from build123d import *

# Parameters (mm, degrees)
SKETCH2_W               = 26
SKETCH2_H               = 6.2
BOSS_EXTRUDE1_DEPTH     = 3
SKETCH3_W               = 6.4
SKETCH3_H               = 22.2
BOSS_EXTRUDE2_DEPTH     = 13.4
SKETCH4_W               = 9
SKETCH4_H               = 5
CUT_EXTRUDE1_DEPTH      = 27.359248851
FILLET1_R               = 1
CUT_EXTRUDE2_DEPTH      = 25.522846491
CUT_EXTRUDE2_DEPTH_BACK = 25.522846491
SKETCH6_W               = 12.6
SKETCH6_H               = 0.5
SKETCH8_W               = 0.3
SKETCH8_H               = 3.8
BOSS_EXTRUDE4_DEPTH     = 12.9
BOSS_EXTRUDE5_START     = -0.5
BOSS_EXTRUDE5_DEPTH     = 0.7
CUT_EXTRUDE3_DEPTH      = 0.2


with BuildPart() as part:
    # Sketch2 → Boss-Extrude1 (new body)
    with BuildSketch(Plane(origin=(0, 0, 0), x_dir=(1, 0, 0), z_dir=(0, 1, 0))):
        Rectangle(SKETCH2_W, SKETCH2_H)
        with BuildLine():
            Line((-10.4, 1.6), (-9.3, 1.6))
            ThreePointArc((-9.3, 1.6), (-7.7, 0), (-9.3, -1.6))
            Line((-9.3, -1.6), (-10.4, -1.6))
            ThreePointArc((-10.4, -1.6), (-12, 0), (-10.4, 1.6))
        make_face(mode=Mode.SUBTRACT)
        with BuildLine():
            Line((10.4, 1.6), (9.3, 1.6))
            ThreePointArc((9.3, 1.6), (7.7, 0), (9.3, -1.6))
            Line((9.3, -1.6), (10.4, -1.6))
            ThreePointArc((10.4, -1.6), (12, 0), (10.4, 1.6))
        make_face(mode=Mode.SUBTRACT)
    extrude(amount=BOSS_EXTRUDE1_DEPTH)

    # Sketch3 → Boss-Extrude2 (add)
    with BuildSketch(Plane(origin=(0, 0, 0), x_dir=(1, 0, 0), z_dir=(0, 1, 0))):
        with Locations((0, 4.8)):
            Rectangle(SKETCH3_W, SKETCH3_H)
    extrude(amount=BOSS_EXTRUDE2_DEPTH)

    # Sketch4 → Cut-Extrude1 (cut, through all)
    with BuildSketch(Plane(origin=(3.2, 0, 0), x_dir=(0, 0, -1), z_dir=(1, 0, 0))):
        with Locations((11.4, 6.7)):
            Rectangle(SKETCH4_W, SKETCH4_H)
    extrude(amount=-CUT_EXTRUDE1_DEPTH, mode=Mode.SUBTRACT)

    # Fillet1
    fillet1_edges = [part.edges().sort_by_distance(p)[0] for p in [
        (-13, 1.5, -3.1),
        (13, 1.5, -3.1),
        (13, 1.5, 3.1),
        (-13, 1.5, 3.1),
    ]]
    fillet(fillet1_edges, radius=FILLET1_R)

    # Sketch6 → Cut-Extrude2 (cut, two sides: drawn at the far end of the back side and taken through both)
    with BuildSketch(Plane.XY.offset(-CUT_EXTRUDE2_DEPTH_BACK)):
        with Locations((0, 0.25)):
            Rectangle(SKETCH6_W, SKETCH6_H)
    extrude(amount=CUT_EXTRUDE2_DEPTH + CUT_EXTRUDE2_DEPTH_BACK, mode=Mode.SUBTRACT)

    # Sketch8 → Boss-Extrude4 (add)
    with BuildSketch(Plane(origin=(0, 13.4, 0), x_dir=(1, 0, 0), z_dir=(0, 1, 0))):
        with Locations((0, -8.2)):
            Rectangle(SKETCH8_W, SKETCH8_H)
    extrude(amount=-BOSS_EXTRUDE4_DEPTH)

    # Sketch9 → Boss-Extrude5 (add)
    # profile 1 of 4: a face of its own
    with BuildSketch(Plane(origin=(3.2, 0, 0), x_dir=(0, 0, -1), z_dir=(1, 0, 0)).offset(BOSS_EXTRUDE5_START)):
        with BuildLine():
            Line((-6.3, 7.72), (-12.2, 7.72))
            ThreePointArc((-12.2, 7.72), (-12.412132034, 7.807867966), (-12.5, 8.02))
            Line((-12.5, 8.02), (-12.5, 8.42))
            ThreePointArc((-12.5, 8.42), (-12.412132034, 8.632132034), (-12.2, 8.72))
            Line((-12.2, 8.72), (-6.3, 8.72))
            Line((-6.3, 8.72), (-6.3, 7.72))
        make_face()
        with BuildLine():
            Line((-11.9, 8.52), (-10.749572658, 8.52))
            ThreePointArc((-10.749572658, 8.52), (-10.449572658, 8.22), (-10.749572658, 7.92))
            Line((-10.749572658, 7.92), (-11.9, 7.92))
            ThreePointArc((-11.9, 7.92), (-12.2, 8.22), (-11.9, 8.52))
        make_face(mode=Mode.SUBTRACT)
    # profile 2 of 4: a face of its own
    with BuildSketch(Plane(origin=(3.2, 0, 0), x_dir=(0, 0, -1), z_dir=(1, 0, 0)).offset(BOSS_EXTRUDE5_START)):
        with BuildLine():
            Line((-6.3, 10.26), (-12.2, 10.26))
            ThreePointArc((-12.2, 10.26), (-12.412132034, 10.347867966), (-12.5, 10.56))
            Line((-12.5, 10.56), (-12.5, 10.96))
            ThreePointArc((-12.5, 10.96), (-12.412132034, 11.172132034), (-12.2, 11.26))
            Line((-12.2, 11.26), (-6.3, 11.26))
            Line((-6.3, 11.26), (-6.3, 10.26))
        make_face()
        with BuildLine():
            Line((-11.9, 11.06), (-10.749572658, 11.06))
            ThreePointArc((-10.749572658, 11.06), (-10.449572658, 10.76), (-10.749572658, 10.46))
            Line((-10.749572658, 10.46), (-11.9, 10.46))
            ThreePointArc((-11.9, 10.46), (-12.2, 10.76), (-11.9, 11.06))
        make_face(mode=Mode.SUBTRACT)
    # profile 3 of 4: a face of its own
    with BuildSketch(Plane(origin=(3.2, 0, 0), x_dir=(0, 0, -1), z_dir=(1, 0, 0)).offset(BOSS_EXTRUDE5_START)):
        with BuildLine():
            Line((-6.3, 5.18), (-12.2, 5.18))
            ThreePointArc((-12.2, 5.18), (-12.412132034, 5.267867966), (-12.5, 5.48))
            Line((-12.5, 5.48), (-12.5, 5.88))
            ThreePointArc((-12.5, 5.88), (-12.412132034, 6.092132034), (-12.2, 6.18))
            Line((-12.2, 6.18), (-6.3, 6.18))
            Line((-6.3, 6.18), (-6.3, 5.18))
        make_face()
        with BuildLine():
            Line((-11.9, 5.98), (-10.749572658, 5.98))
            ThreePointArc((-10.749572658, 5.98), (-10.449572658, 5.68), (-10.749572658, 5.38))
            Line((-10.749572658, 5.38), (-11.9, 5.38))
            ThreePointArc((-11.9, 5.38), (-12.2, 5.68), (-11.9, 5.98))
        make_face(mode=Mode.SUBTRACT)
    # profile 4 of 4: a face of its own
    with BuildSketch(Plane(origin=(3.2, 0, 0), x_dir=(0, 0, -1), z_dir=(1, 0, 0)).offset(BOSS_EXTRUDE5_START)):
        with BuildLine():
            Line((-6.3, 2.64), (-12.2, 2.64))
            ThreePointArc((-12.2, 2.64), (-12.412132034, 2.727867966), (-12.5, 2.94))
            Line((-12.5, 2.94), (-12.5, 3.34))
            ThreePointArc((-12.5, 3.34), (-12.412132034, 3.552132034), (-12.2, 3.64))
            Line((-12.2, 3.64), (-6.3, 3.64))
            Line((-6.3, 3.64), (-6.3, 2.64))
        make_face()
        with BuildLine():
            Line((-11.9, 3.44), (-10.749572658, 3.44))
            ThreePointArc((-10.749572658, 3.44), (-10.449572658, 3.14), (-10.749572658, 2.84))
            Line((-10.749572658, 2.84), (-11.9, 2.84))
            ThreePointArc((-11.9, 2.84), (-12.2, 3.14), (-11.9, 3.44))
        make_face(mode=Mode.SUBTRACT)
    extrude(amount=-BOSS_EXTRUDE5_DEPTH)

    # Sketch10 → Cut-Extrude3 (cut)
    with BuildSketch(Plane(origin=(0, 0, -15.9), x_dir=(-1, 0, 0), z_dir=(0, 0, -1))):
        Polygon((0, 10.297511632), (-1.041523937, 12.086883848), (1.041523937, 12.086883848), align=None)
        Polygon((1.041523937, 3.034586906), (-1.041523937, 3.034586906), (0, 1.447107426), align=None)
    extrude(amount=-CUT_EXTRUDE3_DEPTH, mode=Mode.SUBTRACT)


solid = part.part
Model file for the job. Use its own axes, mm. A direction names the side the tool comes from. Give positions to 0.01 mm unless a question says otherwise; leave off trailing zeros. Order: outer loops, then holes, each group sorted by start corner. A loop starts at its lowest first (then second) coordinate and runs counter-clockwise, first axis right, second up. Notation, with made-up numbers: M 58,-15 L 112,-15 A32 cw 112,18 Z; hole C -10.75,51.5 d6. An arc over 180 degrees is marked long. Put each result on its own line as item: value. Start each with the question number.
(1) Band-saw the part on C-C on y = 6.75. Give the cut face in (x, z).
(2) Pull direction Y, two halves, no side cores. Call faces 4 (the face through (-10, 1, -1.6)), 5 (the face through (0, 4.2, -11)), 6 (the face through (0, 0.5, -3)): released by +Y, released by -Y, zero draft, split by the parting line, or undercut.
(3) Band-saw the part on D-D on x = -5. Give the cut face in (y, z).
(4) Band-saw the part on A-A on z = -12. Give the cut face in (x, y), then the cut area to 3 significant figures.
(5) Band-saw the part on B-B on z = 0. Give the cut face in (x, y).
(6) Pin check, flat tips, straight feed: pin 1 Ø0.6 at (x, z) = (2.5, 11.5) entering from -Y; pin 2 Ø0.5 at (y, z) = (3, 10.5) entering from -X; pin 3 Ø0.5 at (y, z) = (5.5, 8.5) entering from -X. Stop position of each tip, or through.
(7) Drill centre lines: L1, parallel to X at y = 9, z = 8; L2, parallel to X at y = 10.5, z = -1; L3, parallel to Y at x = 5.75, z = 2. Where is each one in solid material? Low to high. Write a range as [from, to].
(8) Tool access for faces 1 (the face through (-8, 1, 3.1)), 2 (the face through (0, 11, -15.7)), 3 (the face through (10, 1, -1.6)): list every direction of +Z, -Z, +X, -X, +Y, -Y with a clear straight run to the whole face (end or side of a thin tool).
Results below:
1. outline: M -3.2,-6.9 L 3.2,-6.9 L 3.2,6.3 L 0.15,6.3 L 0.15,10.1 L -0.15,10.1 L -0.15,6.3 L -3.2,6.3 Z
2. face 4: zero draft
2. face 5: undercut
2. face 6: released by -Y
3. outline: M 0.5,-3.1 L 3,-3.1 L 3,3.1 L 0.5,3.1 Z
4. outline: M -3.2,0.5 L 3.2,0.5 L 3.2,4.2 L -3.2,4.2 Z; M -3.2,9.2 L 3.2,9.2 L 3.2,13.4 L -3.2,13.4 Z
4. area: 50.6 mm2
5. outline: M -13,0 L -12,0 L -12,3 L -13,3 Z; M -7.7,0 L -6.3,0 L -6.3,0.5 L 6.3,0.5 L 6.3,0 L 7.7,0 L 7.7,3 L 3.2,3 L 3.2,13.4 L -3.2,13.4 L -3.2,3 L -7.7,3 Z; M 12,0 L 13,0 L 13,3 L 12,3 Z
6. pin 1: stops at y = 2.64
6. pin 2: stops at x = 2
6. pin 3: stops at x = -0.15
7. L1: x = [-0.15, 0.15]
7. L2: x = [-3.2, 3.2]
7. L3: y = [0.5, 3]
8. face 1: +Z, -X, +Y, -Y
8. face 2: -Z
8. face 3: +Y, -Y
